Answer from the drawing. Dimensions are ordinates in mm from the lowest x, y and z of the part. Round coordinates to 2 decimals unless told otherwise and drop trailing zeros. Write each loop counter-clockwise with the first axis right and the second up, starting at its lowest first coordinate (ties: lowest second). Pieces come first, ordered by that corner, then holes.
1. Straight lines are drawn through the part: probe 1 along X at (y, z) = (1.5, 280.5); probe 2 along X at (y, z) = (7.75, 244). For each, find the intervals that lie inside material, in ascending order.
2. Find section C-C (z = 233). Write down the section's boundary in (x, y), and give its area (3 significant figures).
3. Find section B-B (x = 70). Write down the section's boundary in (y, z).
4. Flat-ended cylindrical pins translate along their axes: pin 1 Ø4 at (x, z) = (142, 58.5) entering from -Y; pin 2 Ø1 at (y, z) = (3.5, 233) entering from -X; pin 3 Ø1 at (y, z) = (4.5, 245.5) entering from -X. Find the tip coordinate at first contact, or state that the pin passes through.
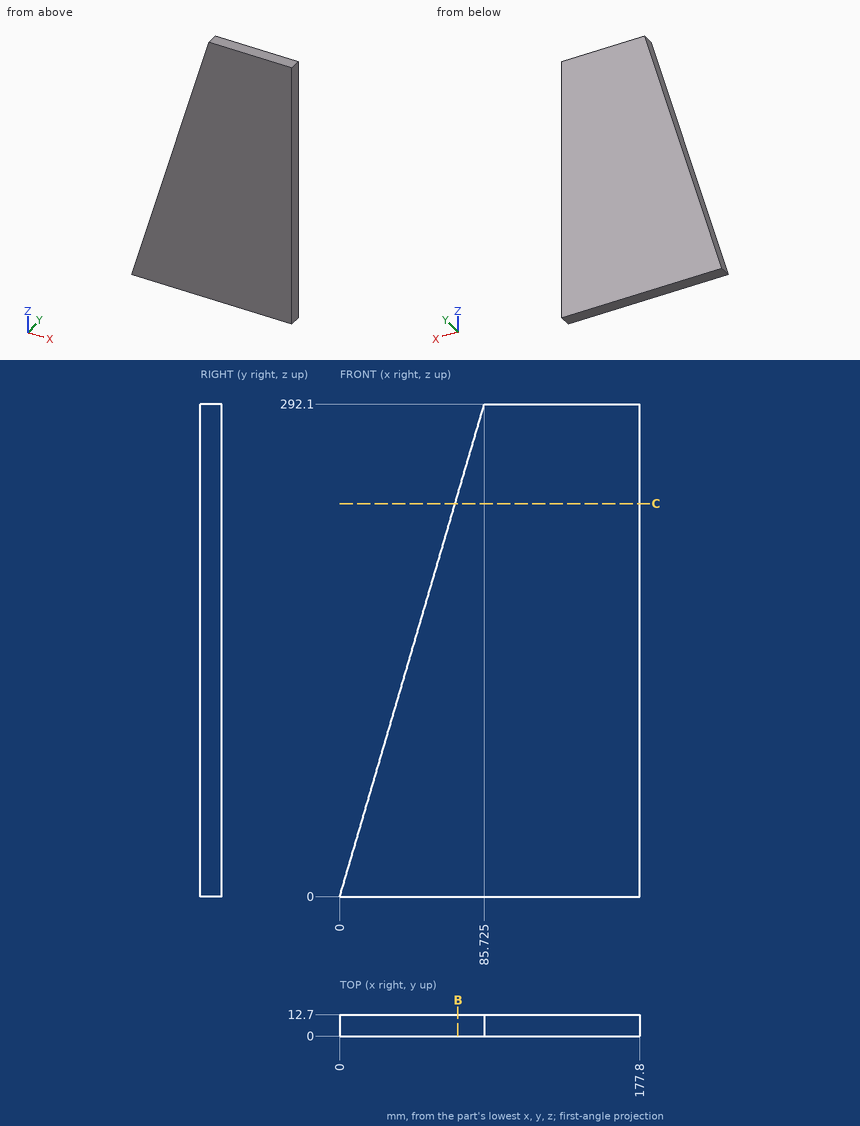
Worked answers:
1. probe 1: x = 82.32 to 177.8
1. probe 2: x = 71.61 to 177.8
2. outline: (68.38, 0) - (177.8, 0) - (177.8, 12.7) - (68.38, 12.7) - close
2. area: 1,390 mm2
3. outline: (0, 0) - (12.7, 0) - (12.7, 238.52) - (0, 238.52) - close
4. pin 1: stops at y = 0
4. pin 2: stops at x = 68.23
4. pin 3: stops at x = 71.9
